Design review of the part built by this model. Coordinates are the model's own, in mm. Face numbers are marked on the shaded views. A direction names the side the tool comes from. Coordinates: 2 decimals unless noted, no trailing zeros. Loops run counter-clockwise (first coordinate to the right, second up) from the corner with the lowest first, then second, coordinate; pieces in that order, holes last. Notation, with made-up numbers: M 7.5,35 L 20.5,35 A18 ccw 20.5,57 Z; hole C 79,81 d6. An arc over 180 degrees is marked long. Answer as a JSON object with one key per item and string values. Group by question number.
1. Consider section A-A (x = 16.5). State the section outline as (y, z) points, then the cut area to 3 significant figures.
2. Draft analysis for pull direction Z (two halves, no side actions). For the marked faces 6, 7 and 8, state which applies: +Z half, -Z half, draft (parallel to the pull), parting line (faces both ways), or undercut.
3. Insertion check: pin 1 (1 mm diameter, centred on x = -21, y = -12, fed in from -Z); pin 2 (18 mm diameter, centred on x = 9, y = -1.5, fed in from -Z); pin 3 (10 mm diameter, centred on x = 34, z = 33.5, fed in from -Y); pin 4 (3.5 mm diameter, centred on x = -13.5, z = 7, fed in from +Y). Each pin has a flat end and moves straight along its axis. Give the tip position at first contact, or say it passes through.
4. Consider section C-C (y = -5). Count the separate pieces of the cut face and the enclosed holes in it, then the cut area to 3 significant figures.
5. Consider section B-B (z = 24). State the section outline as (x, y) points.
6. Machinability: for the marked faces 1, 2, 3, 4 and 5, which of the approach directions +Z, -Z, +X, -X, +Y, -Y give a long, thin tool a straight path to every point of the face, cutting with its end or side? Answer none if there is none.
7. Consider section D-D (x = 0). State the section outline as (y, z) points.
8. To check wall thickness, follow probe 1 along Z at (x, y) = (-8.5, 17); probe 2 along Y at (x, z) = (10, 5); probe 3 along Z at (x, y) = (0, 19.5). State the ranges of each line that lie inside material, in increasing order.
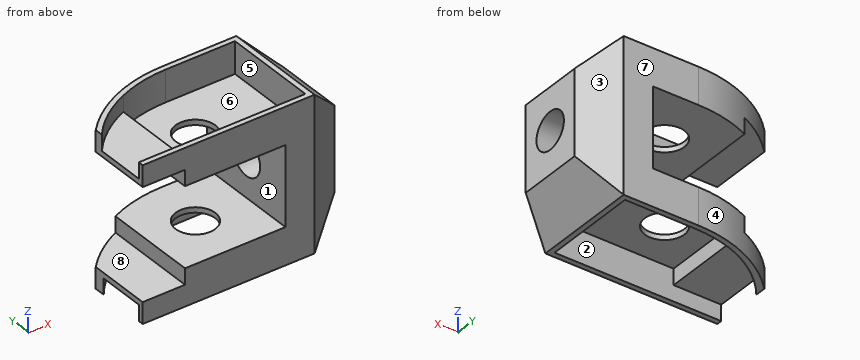
from build123d import *

# Parameters (mm, degrees)
SKETCH1_R           = 7.5
BOSS_EXTRUDE1_DEPTH = 58
SKETCH2_W           = 38
SKETCH2_H           = 30
CUT_EXTRUDE1_DEPTH  = 58
SKETCH3_W           = 16
SKETCH3_H           = 6
CUT_EXTRUDE2_DEPTH  = 58
CUT_EXTRUDE3_DEPTH  = 58
SKETCH5_R           = 7
CUT_EXTRUDE4_DEPTH  = 58
CUT_EXTRUDE5_DEPTH  = 12
CUT_EXTRUDE6_DEPTH  = 6
CUT_EXTRUDE7_DEPTH  = 12
CUT_EXTRUDE8_DEPTH  = 6


with BuildPart() as part:
    # Sketch1 → Boss-Extrude1 (new body)
    with BuildSketch(Plane.XY):
        with BuildLine():
            Line((-34, 5), (-34, -19))
            Line((-34, -19), (31, -19))
            Line((31, -19), (43.990381057, -11.5))
            Line((43.990381057, -11.5), (43.990381057, 13.5))
            Line((43.990381057, 13.5), (31, 21))
            Line((31, 21), (2.66060556, 21))
            ThreePointArc((2.66060556, 21), (-17.33939444, 16.82575695), (-34, 5))
        make_face()
        with Locations(Location((0, 0, 0), (0, 0, 180))):
            Circle(SKETCH1_R, mode=Mode.SUBTRACT)
    extrude(amount=BOSS_EXTRUDE1_DEPTH)

    # Sketch2 → Cut-Extrude1 (cut)
    with BuildSketch(Plane(origin=(0, 21, 0), x_dir=(1, 0, 0), z_dir=(0, 1, 0))):
        with Locations((1, -29)):
            Rectangle(SKETCH2_W, SKETCH2_H)
    extrude(amount=-CUT_EXTRUDE1_DEPTH, mode=Mode.SUBTRACT)

    # Sketch3 → Cut-Extrude2 (cut)
    with BuildSketch(Plane(origin=(0, 21, 0), x_dir=(1, 0, 0), z_dir=(0, 1, 0))):
        with Locations((-26, -11)):
            Rectangle(SKETCH3_W, SKETCH3_H)
        with Locations((-26, -47)):
            Rectangle(SKETCH3_W, SKETCH3_H)
    extrude(amount=-CUT_EXTRUDE2_DEPTH, mode=Mode.SUBTRACT)


with BuildPart() as body_2:
    # of the pieces the cut leaves, the one that is kept (cut_extrude2_keep)
    add(part.part.solids().sort_by_distance((-34, 5, 0))[0])

    # Sketch4 → Cut-Extrude3 (cut)
    with BuildSketch(Plane(origin=(0, 21, 0), x_dir=(1, 0, 0), z_dir=(0, 1, 0))):
        Polygon((31, 0), (43.990381057, 0), (43.990381057, -12.990381057), align=None)
        Polygon((43.990381057, -58), (43.990381057, -45.009618943), (31, -58), align=None)
    extrude(amount=-CUT_EXTRUDE3_DEPTH, mode=Mode.SUBTRACT)

    # Sketch5 → Cut-Extrude4 (cut)
    with BuildSketch(Plane(origin=(43.990381057, 0, 0), x_dir=(0, 0, -1), z_dir=(1, 0, 0))):
        with Locations(Location((-29, 1, 0), (0, 0, 90))):
            Circle(SKETCH5_R)
    extrude(amount=-CUT_EXTRUDE4_DEPTH, mode=Mode.SUBTRACT)

    # Sketch8 → Cut-Extrude5 (cut)
    with BuildSketch(Plane.XY.offset(58)):
        with BuildLine():
            Line((-16, 15.224221872), (-16, -17))
            Line((-16, -17), (29, -17))
            Line((29, -17), (29, 19))
            Line((29, 19), (2.66060556, 19))
            ThreePointArc((2.66060556, 19), (-6.858778616, 18.046586751), (-16, 15.224221872))
        make_face()
    extrude(amount=-CUT_EXTRUDE5_DEPTH, mode=Mode.SUBTRACT)

    # Sketch10 → Cut-Extrude6 (cut)
    with BuildSketch(Plane.XY.offset(58)):
        with BuildLine():
            Line((-16, -17), (-16, 15.224221872))
            ThreePointArc((-16, 15.224221872), (-25.82281671, 9.672366481), (-34, 1.897760392))
            Line((-34, 1.897760392), (-34, -17))
            Line((-34, -17), (-16, -17))
        make_face()
    extrude(amount=-CUT_EXTRUDE6_DEPTH, mode=Mode.SUBTRACT)

    # Sketch11 → Cut-Extrude7 (cut)
    with BuildSketch(Plane(origin=(0, 0, 0), x_dir=(-1, 0, 0), z_dir=(0, 0, -1))):
        with BuildLine():
            Line((16, 15.224221872), (16, -17))
            Line((16, -17), (-29, -17))
            Line((-29, -17), (-29, 19))
            Line((-29, 19), (-2.66060556, 19))
            ThreePointArc((-2.66060556, 19), (6.858778616, 18.046586751), (16, 15.224221872))
        make_face()
    extrude(amount=-CUT_EXTRUDE7_DEPTH, mode=Mode.SUBTRACT)

    # Sketch12 → Cut-Extrude8 (cut)
    with BuildSketch(Plane(origin=(0, 0, 0), x_dir=(-1, 0, 0), z_dir=(0, 0, -1))):
        with BuildLine():
            Line((16, 15.224221872), (16, -17))
            Line((16, -17), (34, -17))
            Line((34, -17), (34, 0.945438982))
            ThreePointArc((34, 0.945438982), (25.900918774, 9.220539125), (16, 15.224221872))
        make_face()
    extrude(amount=-CUT_EXTRUDE8_DEPTH, mode=Mode.SUBTRACT)


solid = body_2.part
Findings below:
{
 "1": {"outline": "M -19,0 L -17,0 L -17,12 L 19,12 L 19,0 L 21,0 L 21,14 L -19,14 Z; M -19,44 L 21,44 L 21,58 L 19,58 L 19,46 L -17,46 L -17,58 L -19,58 Z", "area": "256 mm^2"},
 "2": {"face 6": "+Z half", "face 7": "draft", "face 8": "undercut"},
 "3": {"pin 1": "stops at z = 6", "pin 2": "stops at z = 12", "pin 3": "stops at y = -19", "pin 4": "stops at y = 18.88"},
 "4": {"separate pieces": "4", "enclosed holes": "0", "area": "1,030 mm^2"},
 "5": {"outline": "M 20,-19 L 31,-19 L 43.99,-11.5 L 43.99,-3.9 L 20,-3.9 Z; M 20,5.9 L 43.99,5.9 L 43.99,13.5 L 31,21 L 20,21 Z"},
 "6": {"face 1": "-X, +Y, -Y", "face 2": "-Z", "face 3": "+Z, -Z, +X, +Y", "face 4": "+Z, -Z, -X, +Y", "face 5": "+Z"},
 "7": {"outline": "M -19,0 L -17,0 L -17,12 L -7.5,12 L -7.5,14 L -19,14 Z; M -19,44 L -7.5,44 L -7.5,46 L -17,46 L -17,58 L -19,58 Z; M 7.5,12 L 18.93,12 L 18.93,0 L 20.93,0 L 20.93,14 L 7.5,14 Z; M 7.5,44 L 20.93,44 L 20.93,58 L 18.93,58 L 18.93,46 L 7.5,46 Z"},
 "8": {"probe 1": "z = 12 to 14, 44 to 46", "probe 2": "y = -19 to -17, 19 to 21", "probe 3": "z = 0 to 14, 44 to 58"}
}
